Design review of the part built by this model. Coordinates are the model's own, in mm. A direction names the side the tool comes from. Give positions to 0.01 mm unless a question says otherwise; leave off trailing zeros. Loops run counter-clockwise (first coordinate to the right, second up) from the corner with the lowest first, then second, coordinate; pieces in that order, holes last.
from build123d import *

# Parameters (mm, degrees)
SKETCH2_R                = 80
SKETCH2_R_2              = 7.5
BOSS_EXTRUDE1_DEPTH      = 200
BOSS_EXTRUDE2_DEPTH      = 300
BOSS_EXTRUDE2_DEPTH_BACK = 20
SKETCH2_2_R              = 7.5
FILLET1_R                = 20
BOSS_EXTRUDE3_DEPTH      = 10
CUT_EXTRUDE1_DEPTH       = 10
BOSS_EXTRUDE4_REACH      = 355.977
BOSS_EXTRUDE4_END_RADIUS = 80


with BuildPart() as part:
    # Sketch2 → Boss-Extrude1 (new body)
    with BuildSketch(Plane(origin=(0, 0, 0), x_dir=(1, 0, 0), z_dir=(0, 1, 0))):
        with Locations(Location((0, 0, 0), (0, 0, 270))):
            Circle(SKETCH2_R)
        with Locations(Location((0, 0, 0), (0, 0, 270))):
            Circle(SKETCH2_R_2, mode=Mode.SUBTRACT)
    extrude(amount=BOSS_EXTRUDE1_DEPTH)

    # Sketch2_2 → Boss-Extrude2 (add, two sides: drawn at the far end of the back side and taken through both)
    with BuildSketch(Plane(origin=(0, 0, 0), x_dir=(1, 0, 0), z_dir=(0, 1, 0)).offset(-BOSS_EXTRUDE2_DEPTH_BACK)):
        with Locations(Location((0, 0, 0), (0, 0, 270))):
            Circle(SKETCH2_2_R)
    extrude(amount=BOSS_EXTRUDE2_DEPTH + BOSS_EXTRUDE2_DEPTH_BACK)

    # Fillet1
    fillet1_edges = [part.edges().sort_by_distance(p)[0] for p in [
        (0, 0, -80),
        (0, 200, -80),
    ]]
    fillet(fillet1_edges, radius=FILLET1_R)



with BuildPart() as body_2:
    # Sketch3 → Boss-Extrude3 (new body)
    with BuildSketch(Plane.XY.offset(90)):
        with BuildLine():
            Line((-30, 190), (30, 190))
            ThreePointArc((30, 190), (44.142135624, 184.142135624), (50, 170))
            Line((50, 170), (50, 30))
            ThreePointArc((50, 30), (44.142135624, 15.857864376), (30, 10))
            Line((30, 10), (-30, 10))
            ThreePointArc((-30, 10), (-44.142135624, 15.857864376), (-50, 30))
            Line((-50, 30), (-50, 170))
            ThreePointArc((-50, 170), (-44.142135624, 184.142135624), (-30, 190))
        make_face()
    extrude(amount=BOSS_EXTRUDE3_DEPTH)

    # Sketch3_5 → Cut-Extrude1 (cut)
    with BuildSketch(Plane.XY.offset(90)):
        with BuildLine():
            Line((17.5, 170), (32.5, 170))
            ThreePointArc((32.5, 170), (42.5, 160), (32.5, 150))
            Line((32.5, 150), (17.5, 150))
            ThreePointArc((17.5, 150), (7.5, 160), (17.5, 170))
        make_face()
        with BuildLine():
            Line((15, 87.5), (15, 112.5))
            ThreePointArc((15, 112.5), (25, 122.5), (35, 112.5))
            Line((35, 112.5), (35, 87.5))
            ThreePointArc((35, 87.5), (25, 77.5), (15, 87.5))
        make_face()
        with BuildLine():
            Line((-17.5, 170), (-32.5, 170))
            ThreePointArc((-32.5, 170), (-42.5, 160), (-32.5, 150))
            Line((-32.5, 150), (-17.5, 150))
            ThreePointArc((-17.5, 150), (-7.5, 160), (-17.5, 170))
        make_face()
        with BuildLine():
            Line((17.5, 30), (32.5, 30))
            ThreePointArc((32.5, 30), (42.5, 40), (32.5, 50))
            Line((32.5, 50), (17.5, 50))
            ThreePointArc((17.5, 50), (7.5, 40), (17.5, 30))
        make_face()
        with BuildLine():
            Line((-17.5, 30), (-32.5, 30))
            ThreePointArc((-32.5, 30), (-42.5, 40), (-32.5, 50))
            Line((-32.5, 50), (-17.5, 50))
            ThreePointArc((-17.5, 50), (-7.5, 40), (-17.5, 30))
        make_face()
        with BuildLine():
            Line((-15, 87.5), (-15, 112.5))
            ThreePointArc((-15, 112.5), (-25, 122.5), (-35, 112.5))
            Line((-35, 112.5), (-35, 87.5))
            ThreePointArc((-35, 87.5), (-25, 77.5), (-15, 87.5))
        make_face()
    extrude(amount=CUT_EXTRUDE1_DEPTH, mode=Mode.SUBTRACT)


with BuildPart() as part_1:
    add(part.part)

    add(body_2.part)  # Boss-Extrude4 merges body 2
    # Boss-Extrude4: up to this cylinder (the profile starts outside it)
    boss_extrude4_end = Plane(origin=(0, 100, 0), z_dir=(0, -1, 0)) * Cylinder(BOSS_EXTRUDE4_END_RADIUS, 872.954, mode=Mode.PRIVATE)
    # Sketch6 → Boss-Extrude4 (add, up to the surface)
    with BuildSketch(Plane.XY.offset(90), mode=Mode.PRIVATE) as boss_extrude4_sk1:
        Polygon((-45, 75), (-45, 55), (45, 55), (45, 75), (12.5, 75), (12.5, 125), (45, 125), (45, 145), (-45, 145), (-45, 125), (-12.5, 125), (-12.5, 75), align=None)
    boss_extrude4_tool1 = extrude(boss_extrude4_sk1.sketch, amount=-BOSS_EXTRUDE4_REACH, mode=Mode.PRIVATE) - boss_extrude4_end
    add(boss_extrude4_tool1.solids().sort_by_distance((0, 100, 90))[0])


solid = part_1.part
Q1. Take a section at D-D (y = 236). Give the boundary of the cut face in (x, z).
Results:
outline: circle Ø15 at (0, 0)
Q2. Take a section at B-B (y = 84). Give the boundary of the cut face in (x, z), plus the area to 3 significant figures.
Results:
outline: (-50, 90) - (-34.37, 90) - (-34.37, 100) - (-50, 100) - close; (-15.63, 90) - (-12.5, 90) - (-12.5, 79.02) arc R80 ccw (long way) to (12.5, 79.02) - (12.5, 90) - (15.63, 90) - (15.63, 100) - (-15.63, 100) - close; (34.37, 90) - (50, 90) - (50, 100) - (34.37, 100) - close
area: 21,000 mm2
Q3. Wall thickness on line 1 (Y direction, x = 39.5, z = 84.5); line 2 (Z direction, x = 0.5, y = 44); line 3 (Y direction, x = 10.5, z = -35): over which ranges is each line inside the solid? List them lowest first.
Results:
line 1: y = 55 to 75, 125 to 145
line 2: z = -80 to 80, 90 to 100
line 3: y = 0 to 200
Q4. Insertion check: pin 1 (8 mm diameter, centred on x = 28, z = 96.5, fed in from -Y); pin 2 (3 mm diameter, centred on y = 114.5, z = 43, fed in from -X); pin 3 (10 mm diameter, centred on x = -4, z = 61, fed in from +Y). Each pin has a flat end and moves straight along its axis. Give the tip position at first contact, or say it passes through.
Results:
pin 1: stops at y = 10
pin 2: stops at x = -68.39
pin 3: stops at y = 200
Q5. Take a section at A-A (y = 160). Give the boundary of the cut face in (x, z), plus the area to 3 significant figures.
Results:
outline: circle Ø160 at (0, 0); (-50, 90) - (-42.5, 90) - (-42.5, 100) - (-50, 100) - close; (-7.5, 90) - (7.5, 90) - (7.5, 100) - (-7.5, 100) - close; (42.5, 90) - (50, 90) - (50, 100) - (42.5, 100) - close
area: 20,400 mm2
Q6. Tool access review of faces 3 (the face through (50, 101, 95)), 4 (the face through (-44.297, 183.986, 94.93)), 5 (the face through (-33, 125, 81)), 6 (the face through (-1, 55, 84)): name each direction out of +Z, -Z, +X, -X, +Y, -Y from which nothing blocks a thin tool from reaching the whole face with its end or side.
Results:
face 3: +Z, +X, +Y, -Y
face 4: +Z, -X, +Y
face 5: -X
face 6: -Y
Q7. Draft analysis for pull direction Z (two halves, no side actions). For faces 1 (the face through (-25.2, 77.5, 94.9)), 2 (the face through (12.5, 100, 85)), state which applies: pulls with the +Z half, pulls with the -Z half, needs draft (parallel to the pull), parting line crosses it, or undercut.
Results:
face 1: needs draft
face 2: undercut
Q8. Take a section at C-C (z = 0). Give the boundary of the cut face in (x, y).
Results:
outline: (-80, 20) arc R20 ccw to (-60, 0) - (-7.5, 0) - (-7.5, -20) - (7.5, -20) - (7.5, 0) - (60, 0) arc R20 ccw to (80, 20) - (80, 180) arc R20 ccw to (60, 200) - (7.5, 200) - (7.5, 300) - (-7.5, 300) - (-7.5, 200) - (-60, 200) arc R20 ccw to (-80, 180) - close
